from build123d import *

# Parameters (mm, degrees)
SKETCH1_W                       = 184
SKETCH1_H                       = 64
SKETCH1_W_2                     = 180
SKETCH1_H_2                     = 60
EXTRUDE_THIN1_DEPTH             = 30
SKETCH3_W                       = 184
SKETCH3_H                       = 64
BOSS_EXTRUDE1_DEPTH             = 2
SKETCH4_W                       = 174.419493498
SKETCH4_H                       = 4
CUT_EXTRUDE1_DEPTH              = 5
SKETCH5_W                       = 40.195784268
SKETCH5_H                       = 59.069599678
CUT_EXTRUDE2_DEPTH              = 15
SKETCH6_W                       = 44.195784268
SKETCH6_H                       = 67.776893145
SKETCH6_W_2                     = 40.195784268
SKETCH6_H_2                     = 63.776893145
EXTRUDE_THIN2_DEPTH             = 35
EXTRUDE_THIN2_DIRECTION_2_REACH = 118.55
SKETCH7_W                       = 128.018506196
SKETCH7_H                       = 58.604777903
CUT_EXTRUDE3_DEPTH              = 85
SKETCH8_W                       = 13
SKETCH8_H                       = 30
CUT_EXTRUDE4_DEPTH              = 85
SKETCH9_W                       = 44.195784268
SKETCH9_H                       = 65.776893145
BOSS_EXTRUDE2_DEPTH             = 2
SKETCH13_W                      = 20.06
SKETCH13_H                      = 40.06
CUT_EXTRUDE6_DEPTH              = 10
SKETCH18_R                      = 2.03
CUT_EXTRUDE8_DEPTH              = 10
SKETCH19_W                      = 50
SKETCH19_H                      = 40
CUT_EXTRUDE9_DEPTH              = 10
SKETCH20_R                      = 2.03
CUT_EXTRUDE10_DEPTH             = 10
SKETCH21_W                      = 64
SKETCH21_H                      = 32
CUT_EXTRUDE11_DEPTH             = 217


with BuildPart() as part:
    # Sketch1 → Extrude-Thin1 (new body)
    with BuildSketch(Plane(origin=(0, 0, 0), x_dir=(1, 0, 0), z_dir=(0, 1, 0))):
        Rectangle(SKETCH1_W, SKETCH1_H)
        Rectangle(SKETCH1_W_2, SKETCH1_H_2, mode=Mode.SUBTRACT)
    extrude(amount=EXTRUDE_THIN1_DEPTH)

    # Sketch3 → Boss-Extrude1 (add)
    with BuildSketch(Plane(origin=(0, 30, 0), x_dir=(1, 0, 0), z_dir=(0, 1, 0))):
        Rectangle(SKETCH3_W, SKETCH3_H)
    extrude(amount=BOSS_EXTRUDE1_DEPTH)

    # Sketch4 → Cut-Extrude1 (cut)
    with BuildSketch(Plane(origin=(0, 32, 0), x_dir=(1, 0, 0), z_dir=(0, 1, 0))):
        with Locations((0, -2)):
            Rectangle(SKETCH4_W, SKETCH4_H)
    extrude(amount=-CUT_EXTRUDE1_DEPTH, mode=Mode.SUBTRACT)

    # Sketch5 → Cut-Extrude2 (cut)
    with BuildSketch(Plane.XY.offset(32)):
        with Locations((0, 16)):
            Rectangle(SKETCH5_W, SKETCH5_H)
    extrude(amount=-CUT_EXTRUDE2_DEPTH, mode=Mode.SUBTRACT)

    # Sketch6 → Extrude-Thin2 (add)
    with BuildSketch(Plane.XY.offset(32)):
        with Locations((0, 31.888446573)):
            Rectangle(SKETCH6_W, SKETCH6_H)
        with Locations((0, 31.888446573)):
            Rectangle(SKETCH6_W_2, SKETCH6_H_2, mode=Mode.SUBTRACT)
    extrude(amount=EXTRUDE_THIN2_DEPTH)

    # Extrude-Thin2 direction 2: up to this face of the body (flat: up to its plane)
    extrude_thin2_direction_2_end = Plane(part.part.faces().sort_by_distance((0, 31, 17))[0])
    # Sketch6 → Extrude-Thin2 direction 2 (add, up to the picked face)
    with BuildSketch(Plane.XY.offset(32), mode=Mode.PRIVATE) as extrude_thin2_direction_2_sk1:
        with Locations((0, 31.888446573)):
            Rectangle(SKETCH6_W, SKETCH6_H)
        with Locations((0, 31.888446573)):
            Rectangle(SKETCH6_W_2, SKETCH6_H_2, mode=Mode.SUBTRACT)
    extrude_thin2_direction_2_tool1 = split(extrude(extrude_thin2_direction_2_sk1.sketch, amount=-EXTRUDE_THIN2_DIRECTION_2_REACH, mode=Mode.PRIVATE), bisect_by=extrude_thin2_direction_2_end, keep=Keep.BOTH, mode=Mode.PRIVATE)
    add(extrude_thin2_direction_2_tool1.solids().sort_by(Axis((0, -1.190866, 32), (0, 0, -1)))[0])

    # Sketch7 → Cut-Extrude3 (cut)
    with BuildSketch(Plane.XZ):
        with Locations((2.364457898, 44.353486129)):
            Rectangle(SKETCH7_W, SKETCH7_H)
    extrude(amount=CUT_EXTRUDE3_DEPTH, mode=Mode.SUBTRACT)

    # Sketch8 → Cut-Extrude4 (cut)
    with BuildSketch(Plane.ZY.offset(22.097892134)):
        with Locations((23.5, 15)):
            Rectangle(SKETCH8_W, SKETCH8_H)
    extrude(amount=-CUT_EXTRUDE4_DEPTH, mode=Mode.SUBTRACT)

    # Sketch9 → Boss-Extrude2 (add)
    with BuildSketch(Plane.XY.offset(67)):
        with Locations((0, 32.888446573)):
            Rectangle(SKETCH9_W, SKETCH9_H)
    extrude(amount=BOSS_EXTRUDE2_DEPTH)

    # Sketch13 → Cut-Extrude6 (cut)
    with BuildSketch(Plane.XY.offset(69)):
        with Locations((0, 30.776893145)):
            Rectangle(SKETCH13_W, SKETCH13_H)
    extrude(amount=-CUT_EXTRUDE6_DEPTH, mode=Mode.SUBTRACT)

    # Sketch18 → Cut-Extrude8 (cut)
    with BuildSketch(Plane.XY.offset(69)):
        with Locations((-5, 6.246893145)):
            Circle(SKETCH18_R)
        with Locations((5, 6.246893145)):
            Circle(SKETCH18_R)
    extrude(amount=-CUT_EXTRUDE8_DEPTH, mode=Mode.SUBTRACT)

    # Sketch19 → Cut-Extrude9 (cut)
    with BuildSketch(Plane.XY.offset(32)):
        with Locations((57.048946067, 0)):
            Rectangle(SKETCH19_W, SKETCH19_H)
    extrude(amount=-CUT_EXTRUDE9_DEPTH, mode=Mode.SUBTRACT)

    # Sketch20 → Cut-Extrude10 (cut)
    with BuildSketch(Plane.XY.offset(69)):
        with Locations((-5, 55.306893145)):
            Circle(SKETCH20_R)
        with Locations((5, 55.306893145)):
            Circle(SKETCH20_R)
    extrude(amount=-CUT_EXTRUDE10_DEPTH, mode=Mode.SUBTRACT)

    # Sketch21 → Cut-Extrude11 (cut)
    with BuildSketch(Plane.ZY.offset(92)):
        with Locations((0, 16)):
            Rectangle(SKETCH21_W, SKETCH21_H)
    extrude(amount=-CUT_EXTRUDE11_DEPTH, mode=Mode.SUBTRACT)


solid = part.part
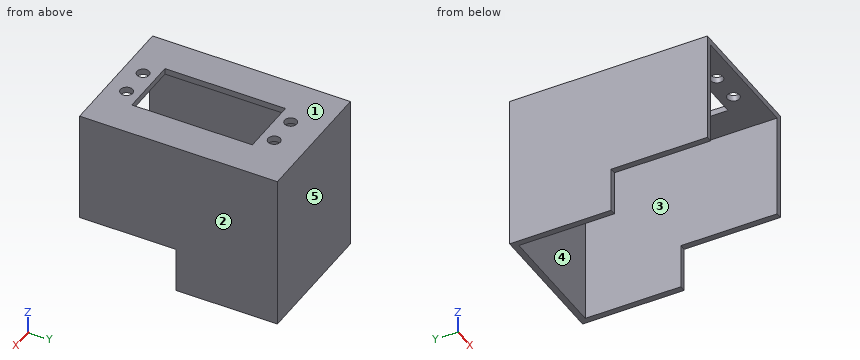
Read the model definition and answer for the solid it produces. Units are mm, in the model's axes. Face numbers are marked on the shaded views. A direction names the side the tool comes from. Give positions to 0.01 mm unless a question says otherwise; leave off trailing zeros. Write each loop counter-clockwise with the first axis right and the second up, starting at its lowest first coordinate (ties: lowest second). Pieces come first, ordered by that corner, then holes. Notation, with made-up numbers: (54.25, -20) - (80.25, -20) arc R31 ccw to (80.25, 19) - close; hole circle Ø6 at (-28, 87.5). An arc over 180 degrees is marked (long way). Return JSON: item names as keys, results as strings.
Q1. A cutting plane is placed at C-C, the plane x = -5. Determine the outline of the cut face in (y, z), and give its area (3 significant figures).
Reply:
{"outline": "(0, 67) - (4.22, 67) - (4.22, 69) - (0, 69) - close; (8.28, 67) - (10.75, 67) - (10.75, 69) - (8.28, 69) - close; (50.81, 67) - (53.28, 67) - (53.28, 69) - (50.81, 69) - close; (57.34, 67) - (63.78, 67) - (63.78, 17) - (65.78, 17) - (65.78, 69) - (57.34, 69) - close", "area": "135 mm²"}
Q2. Consider line 1 along Y through (x, z) = (5, 68.3); line 2 along X through (y, z) = (24, 34); line 3 along Y through (x, z) = (13, 34). Determine where each line is inside the solid, lowest interval first. Write a range as [from, to].
Reply:
{"line 1": "[0, 4.22], [8.28, 10.75], [50.81, 53.28], [57.34, 65.78]", "line 2": "[-22.1, -20.1], [20.1, 22.1]", "line 3": "[63.78, 65.78]"}
Q3. A cutting plane is placed at A-A, the plane x = 8.5. Determine the outline of the cut face in (y, z).
Reply:
{"outline": "(0, 67) - (10.75, 67) - (10.75, 69) - (0, 69) - close; (50.81, 67) - (63.78, 67) - (63.78, 17) - (65.78, 17) - (65.78, 69) - (50.81, 69) - close"}
Q4. A cutting plane is placed at B-B, the plane y = 50. Determine the outline of the cut face in (x, z).
Reply:
{"outline": "(-22.1, 17) - (-20.1, 17) - (-20.1, 67) - (-10.03, 67) - (-10.03, 69) - (-22.1, 69) - close; (10.03, 67) - (20.1, 67) - (20.1, 17) - (22.1, 17) - (22.1, 69) - (10.03, 69) - close"}
Q5. For a pull along X with two mould halves and no side action, classify the marked faces 1, 2 and 3 as released by +X, released by -X, zero draft, split by the parting line, or undercut.
Reply:
{"face 1": "zero draft", "face 2": "released by +X", "face 3": "undercut"}
Q6. For the marked faces 4 and 5, determine the directions among +Z, -Z, +X, -X, +Y, -Y from which every point of the face is accessible in a straight line to the end or side of a thin tool.
Reply:
{"face 4": "-Z, -Y", "face 5": "+Z, -Z, +X, -X, +Y"}
Q7. A cutting plane is placed at D-D, the plane z = 29.5. Determine the outline of the cut face in (x, y), and give its area (3 significant figures).
Reply:
{"outline": "(-22.1, 32) - (-20.1, 32) - (-20.1, 63.78) - (20.1, 63.78) - (20.1, 32) - (22.1, 32) - (22.1, 65.78) - (-22.1, 65.78) - close", "area": "215 mm²"}
Q8. Given P1, Ø12, axis at x = 11, z = 31, coming from the -Y side; P2, Ø2.5, axis at x = -5, y = 55.31, coming from the +Z side; P3, Ø6.5, axis at x = -5, y = 6.25, coming from the -Z side; P4, Ø0.6, axis at x = 21.5, y = 21.5, coming from the -Z side, each flat-ended and moving along its own axis, determine where each tip first touches the part or whether it passes through.
Reply:
{"P1": "y = 63.78", "P2": "through", "P3": "z = 67", "P4": "z = 32"}
